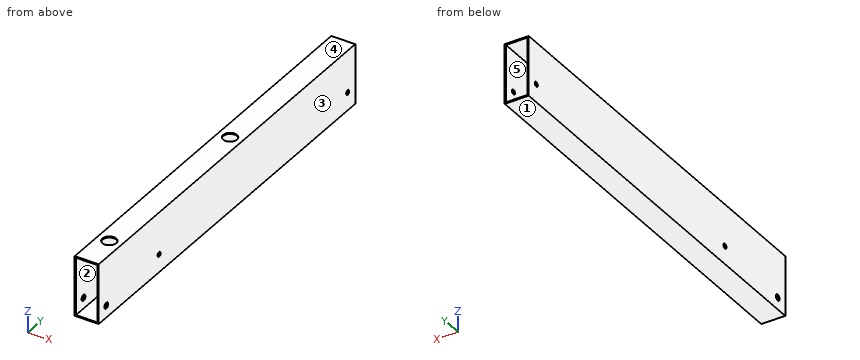
```python
from build123d import *

# Parameters (mm, degrees)
F0_W      = 100
F0_H      = 250
F0_W_2    = 90
F0_H_2    = 240
F1_DEPTH  = 1700
F2_R      = 10
F3_DEPTH  = 100.001
F4_R      = 10
F5_DEPTH  = 100.001
F6_R      = 29
F7_R      = 29
F8_DEPTH  = 5
F9_R      = 12.5
F10_DEPTH = 100.001


# Not quite as in the source:
# - a feature names something its author has since deleted; it is built from what else it names


with BuildPart() as f1:
    # F0 (on Front) → F1 (new body)
    with BuildSketch(Plane.XZ):
        Rectangle(F0_W, F0_H)
        Rectangle(F0_W_2, F0_H_2, mode=Mode.SUBTRACT)
    extrude(amount=F1_DEPTH)

    # F2 (on face) → F3 (cut, through all)
    with BuildSketch(Plane.YZ.offset(50)):
        with Locations((-1300, -50)):
            Circle(F2_R)
    extrude(amount=-F3_DEPTH, mode=Mode.SUBTRACT)

    # F4 (on face) → F5 (cut, through all)
    with BuildSketch(Plane.YZ.offset(50)):
        with Locations((-50, -50)):
            Circle(F4_R)
    extrude(amount=-F5_DEPTH, mode=Mode.SUBTRACT)

    # F6 (on face) + F7 (on face) → F8 (cut, through all)
    with BuildSketch(Plane.XY.offset(125)):
        with Locations((0, -1550)):
            Circle(F6_R)
    with BuildSketch(Plane.XY.offset(125)):
        with Locations((0, -750)):
            Circle(F7_R)
    extrude(amount=-F8_DEPTH, mode=Mode.SUBTRACT)

    # F9 (on face) → F10 (cut, through all)
    with BuildSketch(Plane.YZ.offset(50)):
        with Locations((-1650, -75)):
            Circle(F9_R)
    extrude(amount=-F10_DEPTH, mode=Mode.SUBTRACT)


solid = f1.part
```
Read the model definition and answer for the solid it produces. Units are mm, in the model's axes. Face numbers are marked on the shaded views. A direction names the side the tool comes from. Give positions to 0.01 mm unless a question says otherwise; leave off trailing zeros. Order: outer loops, then holes, each group sorted by start corner. A loop starts at its lowest first (then second) coordinate and runs counter-clockwise, first axis right, second up. Notation, with made-up numbers: (-35, 35) -> (10, 35) arc R4 cw to (10, 40) -> close; hole circle Ø2 at (-26.75, 63.25). An arc over 180 degrees is marked (long way). Write item = value, one per line.
1. A cutting plane is placed at A-A, the plane z = 76.5. Write down the section's boundary in (x, y), and give its area (3 significant figures).
Numbers:
outline = (-50, -1700) -> (-45, -1700) -> (-45, 0) -> (-50, 0) -> close; (45, -1700) -> (50, -1700) -> (50, 0) -> (45, 0) -> close
area = 17,000 mm²
2. A cutting plane is placed at B-B, the plane y = -1192.5. Write down the section's boundary in (x, z).
Numbers:
outline = (-50, -125) -> (50, -125) -> (50, 125) -> (-50, 125) -> close; hole (-45, -120) -> (45, -120) -> (45, 120) -> (-45, 120) -> close
3. Straight lines are drawn through the part: line 1 along Y through (x, z) = (0, 123.9); line 2 along X through (y, z) = (-1547, -56.5); line 3 along Z through (x, y) = (-47.75, -1300). For each, find the intervals that lie inside material, in ascending order.
Numbers:
line_1 = -1700 to -1579, -1521 to -779, -721 to 0
line_2 = -50 to -45, 45 to 50
line_3 = -125 to -60, -40 to 125
4. A cutting plane is placed at C-C, the plane x = 0. Write down the section's boundary in (y, z), and give its area (3 significant figures).
Numbers:
outline = (-1700, -125) -> (0, -125) -> (0, -120) -> (-1700, -120) -> close; (-1700, 120) -> (-1579, 120) -> (-1579, 125) -> (-1700, 125) -> close; (-1521, 120) -> (-779, 120) -> (-779, 125) -> (-1521, 125) -> close; (-721, 120) -> (0, 120) -> (0, 125) -> (-721, 125) -> close
area = 16,400 mm²
5. The mould has two halves that part along Z. Classify the marked faces 1, 2 and 3: +Z half, -Z half, draft (parallel to the pull), parting line (faces both ways), or undercut.
Numbers:
face_1 = -Z half
face_2 = undercut
face_3 = draft
6. For the marked faces 4 and 5, determine the directions among +Z, -Z, +X, -X, +Y, -Y from which every point of the face is accessible in a straight line to the end or side of a thin tool.
Numbers:
face_4 = +Z, +X, -X, +Y, -Y
face_5 = +Y, -Y
7. A cutting plane is placed at D-D, the plane y = -1550. Write down the section's boundary in (x, z).
Numbers:
outline = (-50, -125) -> (50, -125) -> (50, 125) -> (29, 125) -> (29, 120) -> (45, 120) -> (45, -120) -> (-45, -120) -> (-45, 120) -> (-29, 120) -> (-29, 125) -> (-50, 125) -> close
